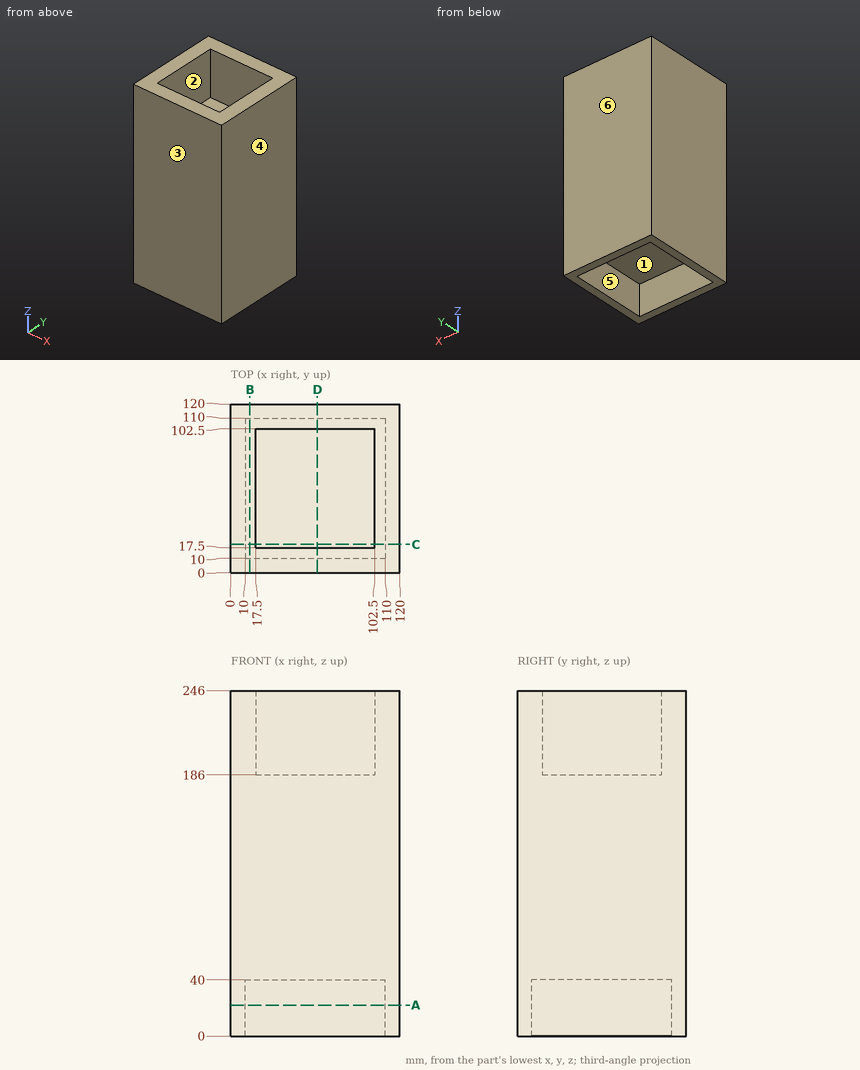
Could you check a few things on this drawing? It's one solid part, dimensions in mm from its lowest x, y, z. A direction names the side the tool comes from. Give positions to 0.01 mm unless a question says otherwise; leave off trailing zeros. Write each loop counter-clockwise with the first axis right and the second up, starting at its lowest first coordinate (ties: lowest second). Pieces come first, ordered by that corner, then holes. Notation, with made-up numbers: M 38,1.25 L 77,1.25 A30 cw 77,37.25 Z; hole C -36,-20 d8. An arc over 180 degrees is marked long. Put each result on its own line as item: value. Start each with the question number.
Item 1: If we section it at B-B, the plane x = 13.5: Write out the boundary of the cut face in (y, z), then the cut area to 3 significant figures.
Item 2: Thinking about a two-plate mould opening in X: for the marked faces 4, 5 and 6, which applies, +X half, -X half, draft (parallel to the pull), parting line (faces both ways), or undercut?
Item 3: I need wall thicknesses on L1, parallel to Y at x = 55, z = 200; L2, parallel to X at y = 102.5, z = 28; L3, parallel to Z at x = 78, y = 108.5. Which ranges of each line are inside material? Lowest first, please. Write a range as from..to.
Item 4: If we section it at C-C, the plane y = 20: Write out the boundary of the cut face in (x, z), then the cut area to 3 significant figures.
Item 5: On a 3-axis mill with a long thin cutter (end or side, diameter ignored), from which of +Z, -Z, +X, -X, +Y, -Y can I reach the whole of each face in a straight line? I mean the marked faces 1, 2 and 3. Say none if no direction works.
Item 6: If we section it at A-A, the plane z = 22: Write out the boundary of the cut face in (x, y).
Item 7: Will these pins go through, and if not, where does the flat tip stop? pin 1 (1.5 mm diameter, centred on x = 63, y = 76, fed in from +Z); pin 2 (8 mm diameter, centred on y = 12.5, z = 139, fed in from -X); pin 3 (8 mm diameter, centred on x = 67, y = 102, fed in from -Z).
Values:
1. outline: M 0,0 L 10,0 L 10,40 L 110,40 L 110,0 L 120,0 L 120,246 L 0,246 Z
1. area: 25,500 mm²
2. face 4: +X half
2. face 5: undercut
2. face 6: draft
3. L1: 0..17.5, 102.5..120
3. L2: 0..10, 110..120
3. L3: 40..246
4. outline: M 0,0 L 10,0 L 10,40 L 110,40 L 110,0 L 120,0 L 120,246 L 102.5,246 L 102.5,186 L 17.5,186 L 17.5,246 L 0,246 Z
4. area: 20,400 mm²
5. face 1: -Z
5. face 2: +Z
5. face 3: +Z, -Z, +X, -X, -Y
6. outline: M 0,0 L 120,0 L 120,120 L 0,120 Z; hole M 10,10 L 110,10 L 110,110 L 10,110 Z
7. pin 1: z = 186
7. pin 2: x = 0
7. pin 3: z = 40
